The model under review builds one solid part; all positions refer to its coordinate system, in mm. Face numbers are marked on the shaded views. A direction names the side the tool comes from. Round coordinates to 2 decimals unless told otherwise and drop trailing zeros. Write each loop counter-clockwise with the first axis right and the second up, starting at its lowest first coordinate (ties: lowest second). Pieces come first, ordered by that corner, then holes. Notation, with made-up numbers: (57, 20) -> (90, 20) arc R22 ccw to (90, 39) -> close; hole circle Ø3 at (-20, 55). An arc over 180 degrees is marked (long way). Return JSON: item names as keys, results as strings. Group by question number.
1. Take a section at B-B, the plane y = -6.5. Write out the cut boundary in (x, z), then the cut area to 3 significant figures.
2. Mouldability with a two-part tool opening along X and no side actions: class the marked faces 1, 2, 3 and 4 as pulls with the +X half, pulls with the -X half, needs draft (parallel to the pull), parting line crosses it, or undercut.
3. For line 1 along X through (y, z) = (-55.5, -33.63); line 2 along X through (y, z) = (-55, -33); line 3 along Y through (x, z) = (2.25, -36), list the stretches that pass through material, from the lowest coordinate up. Write a range as from..to.
4. Tool access review of the marked faces 5 and 6: name each direction out of +Z, -Z, +X, -X, +Y, -Y from which nothing blocks a thin tool from reaching the whole face with its end or side.
5. Take a section at C-C, the plane x = 6. Write out the cut boundary in (y, z), then the cut area to 3 significant figures.
6. Take a section at D-D, the plane z = -25. Write out the cut boundary in (x, y), then the cut area to 3 significant figures.
7. Take a section at A-A, the plane x = 0. Write out the cut boundary in (y, z), then the cut area to 3 significant figures.
8. Clearance check with flat-ended pins moving along their axes: P1, Ø8, axis at x = 1.5, z = -28.5, coming from the +Y side; P2, Ø12, axis at x = 3.5, y = -42.5, coming from the +Z side; P3, Ø4, axis at x = -4.5, y = -22.5, coming from the -Z side; P4, Ø5.5, axis at x = -5, z = -33.63, coming from the -Y side. State where each tip first meets the part, or that it passes through.
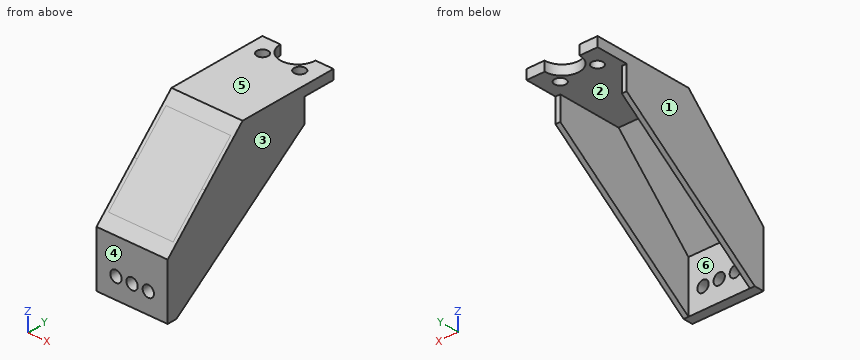
from build123d import *

# Parameters (mm, degrees)
SKETCH1_R               = 1.75
BOSS_EXTRUDE1_DEPTH     = 3
BOSS_EXTRUDE2_DEPTH     = 3
SKETCH4_W               = 40
SKETCH4_H               = 3
BOSS_EXTRUDE3_DEPTH     = 22
SKETCH5_R               = 1.75
CUT_EXTRUDE1_DEPTH      = 10
BOSS_EXTRUDE4_DEPTH     = 1
BOSS_EXTRUDE5_DEPTH     = 22
CUT_EXTRUDE2_DEPTH      = 74.027392121
CUT_EXTRUDE3_DEPTH      = 71.498226928
SKETCH10_R              = 1.75
CUT_EXTRUDE4_DEPTH      = 71.498226928
BOSS_EXTRUDE6_DEPTH     = 1.5
CUT_EXTRUDE5_DEPTH      = 73.589599806
CUT_EXTRUDE5_DEPTH_BACK = 73.589599806


# Read off the part's stored shape, not the designer's step: Boss-Extrude2
with BuildPart() as part:
    # Sketch1 → Boss-Extrude1 (new body)
    with BuildSketch(Plane.XY):
        with BuildLine():
            Line((5.4, 4.03535718), (5.4, 0))
            ThreePointArc((5.4, 0), (0, -5.4), (-5.4, 0))
            Line((-5.4, 0), (-5.4, 4.03535718))
            ThreePointArc((-5.4, 4.03535718), (-7.5, 5.75), (-5.4, 7.46464282))
            Line((-5.4, 7.46464282), (-5.4, 9.583318841))
            ThreePointArc((-5.4, 9.583318841), (0, -11), (5.4, 9.583318841))
            Line((5.4, 9.583318841), (5.4, 7.46464282))
            ThreePointArc((5.4, 7.46464282), (6.856797181, 7.105544171), (7.5, 5.75))
            ThreePointArc((7.5, 5.75), (6.856797181, 4.394455829), (5.4, 4.03535718))
        make_face()
        with Locations((-5.75, -5.75)):
            Circle(SKETCH1_R, mode=Mode.SUBTRACT)
        with Locations((5.75, -5.75)):
            Circle(SKETCH1_R, mode=Mode.SUBTRACT)
    extrude(amount=BOSS_EXTRUDE1_DEPTH)

    # Boss-Extrude2 outline → Boss-Extrude2 (add)
    with BuildSketch(Plane.XY):
        with BuildLine():
            Line((-11, 0), (-11, -57))
            Line((-11, -57), (11, -57))
            Line((11, -57), (11, 0))
            ThreePointArc((11, 0), (0, -11), (-11, 0))
        make_face()
    extrude(amount=BOSS_EXTRUDE2_DEPTH)

    # Sketch4 → Boss-Extrude3 (add)
    with BuildSketch(Plane.ZY.offset(11)):
        with Locations((-20, -55.5)):
            Rectangle(SKETCH4_W, SKETCH4_H)
    extrude(amount=-BOSS_EXTRUDE3_DEPTH)

    # Sketch5 → Cut-Extrude1 (cut)
    with BuildSketch(Plane(origin=(0, -57, 0), x_dir=(-1, 0, 0), z_dir=(0, -1, 0))):
        with Locations(Location((0, 33.63, 0), (0, 0, 90))):
            Circle(SKETCH5_R)
    extrude(amount=-CUT_EXTRUDE1_DEPTH, mode=Mode.SUBTRACT)

    # Sketch6 → Boss-Extrude4 (add)
    with BuildSketch(Plane.ZY.offset(11)):
        Polygon((-20, -54), (0, -34), (0, -54), align=None)
    boss_extrude4 = extrude(amount=-BOSS_EXTRUDE4_DEPTH)

    # Mirror1: Boss-Extrude4 across plane
    add(boss_extrude4.mirror(Plane(origin=(0, 0, 0), x_dir=(0, 0, 1), z_dir=(1, 0, 0))))

    # Sketch7 → Boss-Extrude5 (add, through all)
    with BuildSketch(Plane(origin=(11, 0, 0), x_dir=(0, 0, -1), z_dir=(1, 0, 0))):
        Polygon((0, -30), (24, -54), (19.757359313, -54), (0, -34.242640687), align=None)
    extrude(amount=-BOSS_EXTRUDE5_DEPTH)

    # Sketch8 → Cut-Extrude2 (cut, through all)
    with BuildSketch(Plane(origin=(11, 0, 0), x_dir=(0, 0, -1), z_dir=(1, 0, 0))):
        Polygon((9.878679656, -44.121320344), (22.757359313, -57), (-3, -57), (-3, -31.242640687), align=None)
    extrude(amount=-CUT_EXTRUDE2_DEPTH, mode=Mode.SUBTRACT)

    # Sketch9 → Cut-Extrude3 (cut, through all)
    with BuildSketch(Plane(origin=(0, 0, 0), x_dir=(-1, 0, 0), z_dir=(0, 0, -1))):
        Polygon((-5.4, 0), (-11, 0), (-11, 9.583318841), (11, 9.583318841), (11, 0), align=None)
    extrude(amount=-CUT_EXTRUDE3_DEPTH, mode=Mode.SUBTRACT)

    # Sketch10 → Cut-Extrude4 (cut, through all)
    with BuildSketch(Plane(origin=(0, -57, 0), x_dir=(-1, 0, 0), z_dir=(0, -1, 0))):
        with Locations(Location((5, 33.63, 0), (0, 0, 90))):
            Circle(SKETCH10_R)
        with Locations((-5, 33.63)):
            Circle(SKETCH10_R)
    extrude(amount=-CUT_EXTRUDE4_DEPTH, mode=Mode.SUBTRACT)

    # Sketch11 → Boss-Extrude6 (add)
    with BuildSketch(Plane(origin=(11, 0, 0), x_dir=(0, 0, -1), z_dir=(1, 0, 0))):
        Polygon((0, 0), (40, -54), (40, -57), (22.757359313, -57), (-3, -31.242640687), (-3, 0), align=None)
    boss_extrude6 = extrude(amount=-BOSS_EXTRUDE6_DEPTH)

    # Mirror2: Boss-Extrude6 across plane
    add(boss_extrude6.mirror(Plane(origin=(0, 0, 0), x_dir=(0, 0, 1), z_dir=(1, 0, 0))))

    # Sketch12 → Cut-Extrude5 (cut, two sides: drawn at the far end of the back side and taken through both)
    with BuildSketch(Plane.ZY.offset(-9.5).offset(-CUT_EXTRUDE5_DEPTH_BACK)):
        Polygon((0, 0), (0, -9.949403651), (-10.711431508, -9.949403651), (-10.711431508, 0.731169273), align=None)
    extrude(amount=CUT_EXTRUDE5_DEPTH + CUT_EXTRUDE5_DEPTH_BACK, mode=Mode.SUBTRACT)


solid = part.part
Output:
{
 "1": {"outline": "(-11, 0) -> (-7.33, 0) -> (-7.33, 3) -> (-11, 3) -> close; (-4.17, 0) -> (4.17, 0) -> (4.17, 3) -> (-4.17, 3) -> close; (7.33, 0) -> (11, 0) -> (11, 3) -> (7.33, 3) -> close", "area": "47.0 mm^2"},
 "2": {"face 1": "pulls with the -X half", "face 2": "undercut", "face 3": "pulls with the +X half", "face 4": "needs draft"},
 "3": {"line 1": "x = -11..-6.75, -3.25..-1.75, 1.75..3.25, 6.75..11", "line 2": "x = -11..-6.63, -3.37..-1.63, 1.63..3.37, 6.63..11", "line 3": "y = -57..-54"},
 "4": {"face 5": "+Z, +X, -X, +Y, -Y", "face 6": "-Z, +Y"},
 "5": {"outline": "(-57, -40) -> (-54, -40) -> (-54, -35.07) -> (-57, -35.07) -> close; (-57, -32.19) -> (-54, -32.19) -> (-54, -24) -> (-30, 0) -> (-7.48, 0) -> (-7.48, 3) -> (-31.24, 3) -> (-57, -22.76) -> close; (-4.02, 0) -> (0, 0) -> (0, 3) -> (-4.02, 3) -> close", "area": "228 mm^2"},
 "6": {"outline": "(-11, -57) -> (11, -57) -> (11, -33.75) -> (9.5, -33.75) -> (9.5, -54) -> (-9.5, -54) -> (-9.5, -33.75) -> (-11, -33.75) -> close", "area": "127 mm^2"},
 "7": {"outline": "(-57, -40) -> (-54, -40) -> (-54, -35.38) -> (-57, -35.38) -> close; (-57, -31.88) -> (-54, -31.88) -> (-54, -24) -> (-30, 0) -> (-5.4, 0) -> (-5.4, 3) -> (-31.24, 3) -> (-57, -22.76) -> close", "area": "221 mm^2"},
 "8": {"P1": "stops at y = -54", "P2": "stops at z = -2.26", "P3": "stops at z = 0", "P4": "stops at y = -57"}
}
